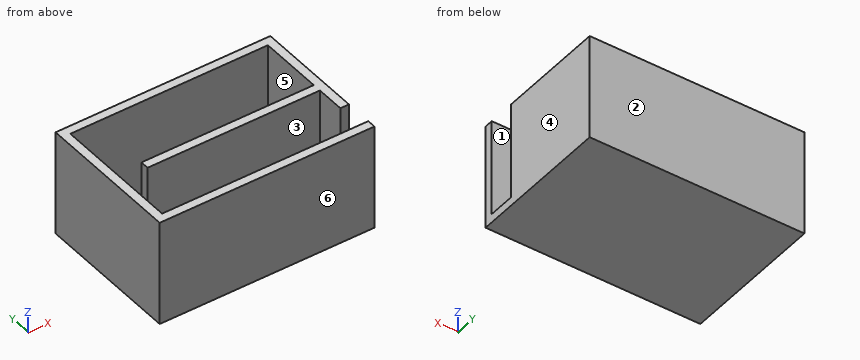
Autodesk Inventor part; units mm, degrees
ref_plane "YZ Plane" through (0, 0, 0) normal (1, 0, 0) x (0, 1, 0)
ref_plane "XZ Plane" through (0, 0, 0) normal (0, 1, 0) x (-1, 0, 0)
ref_plane "XY Plane" through (0, 0, 0) normal (0, 0, 1) x (1, 0, 0)
sketch "Sketch1" plane through (0, 0, 0) normal (0, 0, 1) x (1, 0, 0)
  line L0 (0, 0) -> (400, 0)
  line L1 (400, 0) -> (400, 270)
  line L2 (400, 270) -> (0, 270)
  line L3 (0, 270) -> (0, 0)
  dimension "d0" = 400
  dimension "d1" = 270
extrude "Extrusion1" add sketch "Sketch1" along normal blind 16
sketch "Sketch2" plane through (0, 0, 16) normal (0, 0, 1) x (1, 0, 0)
  line L0 (0, 0) -> (400, 0)
  line L1 (400, 0) -> (400, 270)
  line L2 (400, 270) -> (0, 270)
  line L3 (0, 270) -> (0, 0)
  line L4 (16, 16) -> (384, 16)
  line L5 (384, 16) -> (384, 254)
  line L6 (384, 254) -> (16, 254)
  line L7 (16, 254) -> (16, 16)
  dimension "d4" = 16
  dimension "d5" = 16
  dimension "d6" = 16
  dimension "d7" = 16
extrude "Extrusion2" add sketch "Sketch2" along normal blind 180
sketch "Sketch3" plane through (0, 0, 196) normal (0, 0, 1) x (1, 0, 0)
  line L0 (16, 254) -> (16, 16)
  line L1 (16, 16) -> (384, 16)
  line L2 (384, 16) -> (384, 254)
  line L3 (384, 254) -> (16, 254)
  line L4 (384, 254) -> (384, 16)
  line L5 (400, 0) -> (400, 270)
  line L6 (384, 16) -> (400, 16)
  line L7 (400, 16) -> (400, 66)
  line L8 (400, 66) -> (384, 66)
  line L9 (384, 66) -> (384, 16)
  point P0 (0, 0)
  dimension "d10" = 50
extrude "Extrusion3" cut sketch "Sketch3" against normal blind 180 contours L2 L8 L5 L6
sketch "Sketch4" plane through (0, 0, 196) normal (0, 0, 1) x (1, 0, 0)
  line L0 (16, 254) -> (16, 16)
  line L1 (400, 16) -> (16, 16)
  line L2 (400, 66) -> (400, 16)
  line L3 (384, 66) -> (400, 66)
  line L4 (384, 66) -> (384, 254)
  line L5 (384, 254) -> (16, 254)
  line L6 (384, 66) -> (400, 66)
  line L7 (400, 66) -> (400, 270)
  line L8 (400, 270) -> (0, 270)
  line L9 (0, 270) -> (0, 0)
  line L10 (0, 0) -> (400, 0)
  line L11 (400, 0) -> (400, 16)
  line L12 (400, 16) -> (16, 16)
  line L13 (16, 16) -> (16, 254)
  line L14 (16, 254) -> (384, 254)
  line L15 (384, 254) -> (384, 66)
  line L16 (384, 254) -> (384, 66)
  line L17 (384, 254) -> (62.9229, 254)
  line L18 (62.9229, 254) -> (62.9229, 119)
  line L19 (62.9229, 119) -> (384, 119)
  line L20 (384, 119) -> (384, 254)
  line L21 (384, 254) -> (16, 254)
  line L22 (384, 254) -> (62.9229, 254)
  line L23 (62.9229, 254) -> (62.9229, 135)
  line L24 (62.9229, 135) -> (384, 135)
  line L25 (384, 135) -> (384, 254)
  dimension "d13" = 135
  dimension "d14" = 16
extrude "Extrusion4" add sketch "Sketch4" against normal blind 180 contours L24 L4 L19 L18
properties part number "box"
Here's how the part is built. I have some questions about the finished solid (model axes, mm). Face numbers are marked on the shaded views. A direction names the side the tool comes from. Coordinates: 2 decimals unless noted, no trailing zeros. Loops run counter-clockwise (first coordinate to the right, second up) from the corner with the lowest first, then second, coordinate; pieces in that order, holes last.
1. Imagine slicing it at B-B, the plane x = 240.5. Please give me the cut outline in (y, z).
2. Imagine slicing it at A-A, the plane z = 35. Please give me the cut outline in (x, y), and give its area (3 significant figures).
3. I need wall thicknesses on L1, parallel to Y at x = 188, z = 182; L2, parallel to X at y = 137.5, z = 71.5; L3, parallel to X at y = 52, z = 171. Which ranges of each line are inside material? Lowest first, please.
4. Imagine slicing it at D-D, the plane y = 243.5. Please give me the cut outline in (x, z).
5. Imagine slicing it at C-C, the plane y = 56.5. Please give me the cut outline in (x, z), and give its area (3 significant figures).
6. If we mould it in two halves opening along X, with no side actions, what happens to the marked faces 4, 5 and 6? For each: pulls with the +X half, pulls with the -X half, needs draft (parallel to the pull), parting line crosses it, or undercut.
7. For the marked faces 1, 2 and 3, which set-ups out of +Z, -Z, +X, -X, +Y, -Y let a thin tool reach every point of the face, with its end or its side?
Taken from the geometry:
1. outline: (0, 0) - (270, 0) - (270, 196) - (254, 196) - (254, 16) - (135, 16) - (135, 196) - (119, 196) - (119, 16) - (16, 16) - (16, 196) - (0, 196) - close
2. outline: (0, 0) - (400, 0) - (400, 16) - (16, 16) - (16, 254) - (384, 254) - (384, 135) - (62.92, 135) - (62.92, 119) - (384, 119) - (384, 66) - (400, 66) - (400, 270) - (0, 270) - close
2. area: 24,800 mm2
3. L1: y = 0 to 16, 119 to 135, 254 to 270
3. L2: x = 0 to 16, 384 to 400
3. L3: x = 0 to 16
4. outline: (0, 0) - (400, 0) - (400, 196) - (384, 196) - (384, 16) - (16, 16) - (16, 196) - (0, 196) - close
5. outline: (0, 0) - (400, 0) - (400, 16) - (16, 16) - (16, 196) - (0, 196) - close
5. area: 9,280 mm2
6. face 4: pulls with the +X half
6. face 5: undercut
6. face 6: needs draft
7. face 1: +Z, +X
7. face 2: +Z, -Z, +X, -X, +Y
7. face 3: +Z
